Model file for the job. Use its own axes, mm. Round coordinates to 2 decimals unless told otherwise and drop trailing zeros. Loops run counter-clockwise (first coordinate to the right, second up) from the corner with the lowest first, then second, coordinate; pieces in that order, holes last. Notation, with made-up numbers: M 9,56.5 L 52,56.5 A16 ccw 52,60.5 Z; hole C 31,0 d11. An arc over 180 degrees is marked long. Use a Markdown table: item, result. Add a question column.
Q1. Cut at D-D (x = 61). Give the cut face in (y, z).
Q2. Cut at A-A (x = -16.5). Give the cut face in (y, z).
Q3. Pin check, flat tips, straight feed: pin 1 (1.5 mm diameter, centred on x = 14.5, z = 4, fed in from -Y); pin 2 (0.8 mm diameter, centred on x = 21, z = 4, fed in from +Y); pin 3 (1.3 mm diameter, centred on y = 32.5, z = 3.5, fed in from -X). Stop position of each tip, or through.
Q4. Cut at C-C (y = 4.5). Give the cut face in (x, z), plus the area to 3 significant figures.
Q5. Probe line 1 (Z direction, x = -13.5, y = 63.5); line 2 (Y direction, x = 2, z = 2.7). List the from-to ranges inside material, lowest first. Write a range as from..to.
Q6. Cut at B-B (z = 4.2). State how many separate pieces and enclosed holes the cut face has, plus the area to 3 significant figures.
from build123d import *

# Parameters (mm, degrees)
F0_W      = 146.40107
F0_H      = 148.310445
F1_DEPTH  = 2.54
F4_DEPTH  = 2.54
F6_DEPTH  = 2.54
F8_DEPTH  = 2.54
F9_W      = 4.851737
F9_H      = 18.426374
F10_DEPTH = 2.54
F12_DEPTH = 2.54
F14_DEPTH = 2.54
F15_W     = 1.578693
F15_H     = 13.412963
F16_DEPTH = 2.54
F17_W     = 4.364304
F17_H     = 17.427249
F18_DEPTH = 2.54


with BuildPart() as f1:
    # F0 (on Top) → F1 (new body)
    with BuildSketch(Plane.XY):
        with Locations((-0.210952, 0.137563)):
            Rectangle(F0_W, F0_H)
    extrude(amount=F1_DEPTH)

    # F3 (on offset) → F4 (join)
    with BuildSketch(Plane.XY.offset(2.54)):
        Polygon((-64.964116, 41.773472), (-68.692707, 42.022042), (-68.692707, 22.384809), (-59.246946, 22.384809), align=None)
    extrude(amount=F4_DEPTH)

    # F5 (on offset) → F6 (join)
    with BuildSketch(Plane.XY.offset(2.54)):
        Polygon((-50.52999, 40.857933), (-55.370778, 22.743205), (-47.918595, 22.743205), (-47.918595, 26.920337), (-44.406321, 26.920337), (-44.406321, 36.838796), (-47.918595, 36.838796), (-47.918595, 40.857933), align=None)
    extrude(amount=F6_DEPTH)

    # F7 (on offset) → F8 (join)
    with BuildSketch(Plane.XY.offset(2.54)):
        Polygon((-35.617545, 36.038097), (-39.623722, 36.063977), (-39.623722, 27.117148), (-36.453769, 27.117148), (-36.453769, 22.621898), (-31.509895, 22.621898), (-31.509895, 40.49129), (-35.617545, 40.49129), align=None)
    extrude(amount=F8_DEPTH)

    # F9 (on offset) → F10 (join)
    with BuildSketch(Plane.XY.offset(2.54)):
        with Locations((-17.03154, 31.691134)):
            Rectangle(F9_W, F9_H)
    extrude(amount=F10_DEPTH)

    # F11 (on offset) → F12 (join)
    with BuildSketch(Plane.XY.offset(2.54)):
        Polygon((2.639255, 41.013792), (-2.057669, 40.791102), (-2.057669, 36.814019), (-5.565096, 36.814019), (-5.565096, 33.358328), (-2.61138, 33.358328), (-2.61138, 29.607166), (-5.565096, 29.607166), (-5.565096, 26.148241), (-2.61138, 26.148241), (-2.61138, 22.650495), (6.022215, 22.650495), (6.022215, 36.814019), (2.639255, 36.814019), align=None)
    extrude(amount=F12_DEPTH)

    # F13 (on offset) → F14 (join)
    with BuildSketch(Plane.XY.offset(2.54)):
        Polygon((18.820403, 36.453847), (15.066023, 36.453847), (15.066023, 22.535659), (22.926439, 22.535659), (22.926439, 40.634211), (18.820403, 40.634211), align=None)
    extrude(amount=F14_DEPTH)

    # F15 (on offset) → F16 (join)
    with BuildSketch(Plane.XY.offset(2.54)):
        with Locations((30.708009, 33.6177)):
            Rectangle(F15_W, F15_H)
    extrude(amount=F16_DEPTH)

    # F17 (on offset) → F18 (join)
    with BuildSketch(Plane.XY.offset(2.54)):
        with Locations((40.387601, 31.565268)):
            Rectangle(F17_W, F17_H)
    extrude(amount=F18_DEPTH)


solid = f1.part
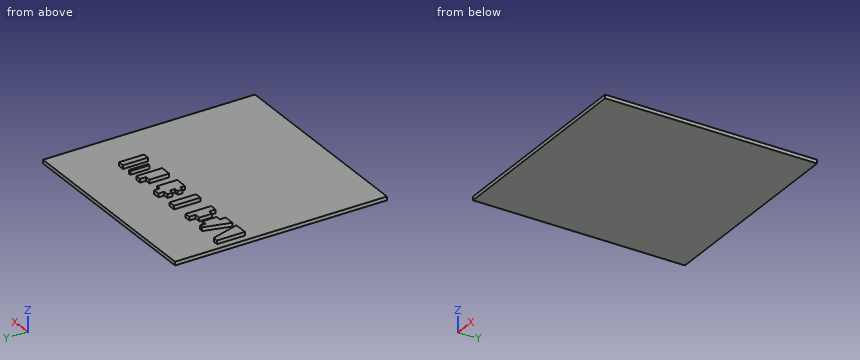
Checked values:
| question | item | result |
|---|---|---|
| 1 | outline | M -74.02,0 L 74.29,0 L 74.29,2.54 L -74.02,2.54 Z |
| 2 | outline | M -74.02,0 L 74.29,0 L 74.29,2.54 L 40.9,2.54 L 40.9,5.08 L 22.48,5.08 L 22.48,2.54 L -74.02,2.54 Z |
| 3 | pin 1 | stops at y = 22.54 |
| 3 | pin 2 | stops at y = 40.63 |
| 3 | pin 3 | stops at x = -68.69 |
| 4 | outline | M -73.41,0 L 72.99,0 L 72.99,2.54 L -73.41,2.54 Z |
| 4 | area | 372 mm^2 |
| 5 | line 1 | z = 0..2.54 |
| 5 | line 2 | y = 22.65..40.98 |
| 6 | separate pieces | 8 |
| 6 | enclosed holes | 0 |
| 6 | area | 842 mm^2 |
